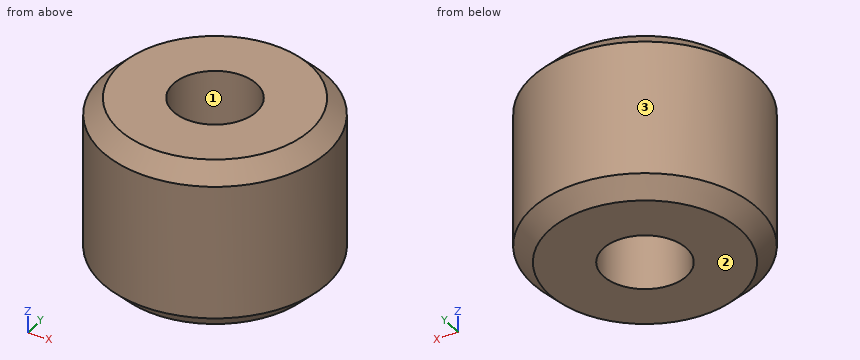
```python
from build123d import *

# Parameters (mm, degrees)
F0_R     = 33.993952
F1_DEPTH = 50.8
F2_SIZE  = 5.08
F3_R     = 12.582727
F4_DEPTH = 76.2


with BuildPart() as f1:
    # F0 (on Top) → F1 (new body)
    with BuildSketch(Plane.XY):
        Circle(F0_R)
    extrude(amount=F1_DEPTH)

    # F2
    f2_edges = [f1.edges().sort_by_distance(p)[0] for p in [
        (-33.993952, 0, 50.8),
        (-33.993952, 0, 0),
    ]]
    chamfer(f2_edges, length=F2_SIZE)

    # F3 (on face) → F4 (cut)
    with BuildSketch(Plane.XY.offset(50.8)):
        Circle(F3_R)
    extrude(amount=-F4_DEPTH, mode=Mode.SUBTRACT)


solid = f1.part
```
CAD build for the part. Positions are in the model's coordinates, mm. Face numbers are marked on the shaded views. Round coordinates to 2 decimals unless told otherwise and drop trailing zeros. Write each loop counter-clockwise with the first axis right and the second up, starting at its lowest first coordinate (ties: lowest second). Pieces come first, ordered by that corner, then holes. Notation, with made-up numbers: (62, 0) - (93, 0) arc R37 ccw to (93, 37) - close; hole circle Ø4 at (25, 51.5). An arc over 180 degrees is marked (long way). Return JSON: item names as keys, results as strings. Group by question number.
Item 1: Flat gauge pins, fed straight in: pin 1 Ø6 at (x, z) = (-24.5, 37.5) entering from -Y; pin 2 Ø5 at (y, z) = (-8.5, 35) entering from -X; pin 3 Ø2 at (x, z) = (-10, 16.5) entering from -Y; pin 4 Ø12 at (x, y) = (3, -5.5) entering from +Z. Where does each tip first touch, or does it go through?
Item 2: Band-saw the part on A-A on x = 0. List the corners of the cut face in (y, z).
Item 3: Probe probe 1 along Y at (x, z) = (0, 37.5); probe 2 along X at (y, z) = (5.5, 2); probe 3 along X at (y, z) = (-4, 20.5). List the from-to ranges inside material, lowest first.
Item 4: Band-saw the part on C-C on z = 31. List the corners of the cut face in (x, y).
Item 5: Mould opens along Y. For the marked faces 1, 2 and 3 say: +Y half, -Y half, draft (parallel to the pull), parting line (faces both ways), or undercut.
Resolved:
{
 "1": {"pin 1": "stops at y = -26.33", "pin 2": "stops at x = -33.46", "pin 3": "stops at y = -32.78", "pin 4": "passes through"},
 "2": {"outline": "(-33.99, 5.08) - (-28.91, 0) - (-12.58, 0) - (-12.58, 50.8) - (-28.91, 50.8) - (-33.99, 45.72) - close; (12.58, 0) - (28.91, 0) - (33.99, 5.08) - (33.99, 45.72) - (28.91, 50.8) - (12.58, 50.8) - close"},
 "3": {"probe 1": "y = -33.99 to -12.58, 12.58 to 33.99", "probe 2": "x = -30.42 to -11.32, 11.32 to 30.42", "probe 3": "x = -33.76 to -11.93, 11.93 to 33.76"},
 "4": {"outline": "circle Ø67.99 at (0, 0); hole circle Ø25.17 at (0, 0)"},
 "5": {"face 1": "undercut", "face 2": "draft", "face 3": "parting line"}
}
